Input: dimensioned drawing with shaded views. Units: mm. Origin: part minimum x, y, z. A direction names the side the tool comes from. Give positions to 0.01 mm unless a question says otherwise; leave off trailing zeros. Order: outer loops, then holes, each group sorted by start corner. A loop starts at its lowest first (then second) coordinate and runs counter-clockwise, first axis right, second up. Notation, with made-up numbers: M 81,3.25 L 86,3.25 A11 ccw 86,12.25 Z; hole C 65,86.5 d4. An arc over 180 degrees is marked long. Answer in a Markdown table with one row per item. Add a question column.
(1) Section query C-C, the plane z = 14. Return loops of the section in (x, y), plus the area to 3 significant figures.
(2) Pin query (flat end, axial travel): P1, Ø4, axis at x = 49.5, z = 19.5, coming from the +Y side; P2, Ø2.5, axis at x = 57.63, y = 57.63, coming from the -Z side; P3, Ø1.9, axis at y = 5, z = 29, coming from the +X side; P4, Ø5, axis at y = 66.5, z = 27, coming from the +X side (1 decimal). Return the tip coordinate at first contact, or that it passes through.
(3) Material intervals for line 1 along Y through (x, z) = (34, 8) (1 decimal); line 2 along Y through (x, z) = (46, 7.5) (1 decimal); line 3 along X through (y, z) = (47, 25.5), sorted ascending.
(4) Mould query, pull axis Y, two halves, no side actions, for the marked faces 4, 5 and 6. Classes: pulls with the +Y half, pulls with the -Y half, needs draft (parallel to the pull), parting line crosses it, or undercut.
(5) Section query A-A, the plane y = 35. Return loops of the section in (x, z), plus the area to 3 significant figures.
(6) Set-up query: the marked faces 1, 2 and 3. Return all of +Z, -Z, +X, -X, +Y, -Y with unobstructed straight access to the full face (end or side cutting, diameter ignored); none if empty.
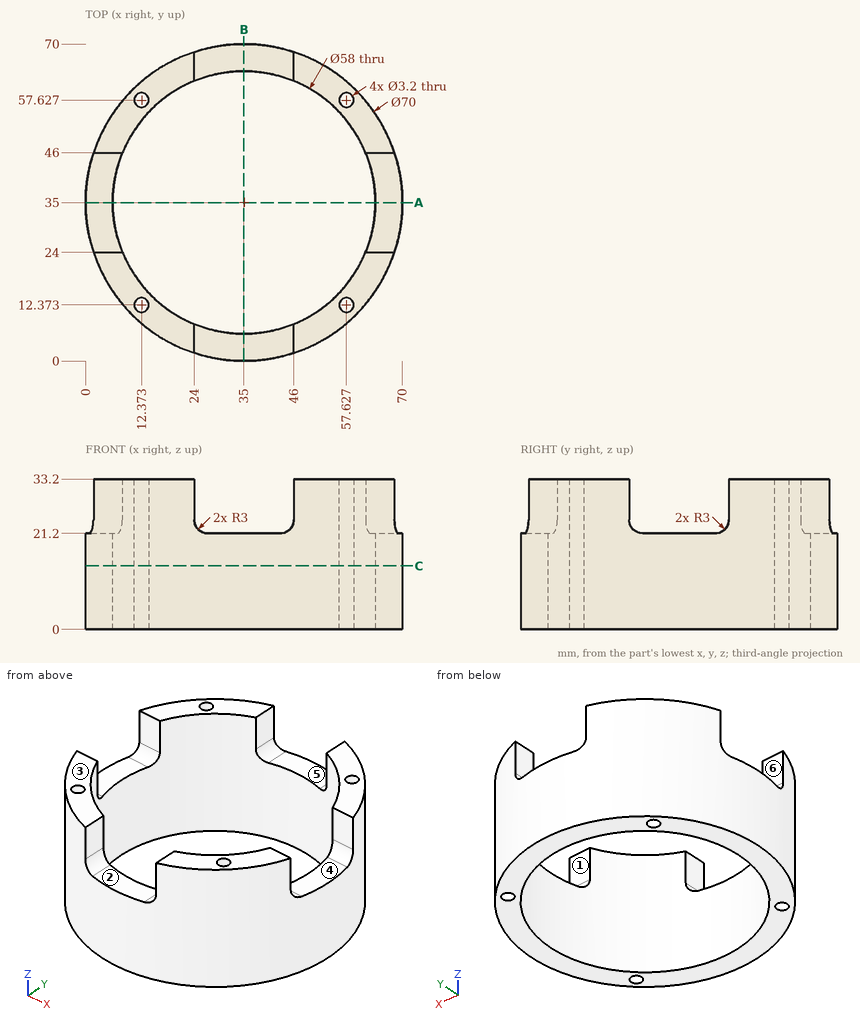
Values follow:
| question | item | result |
|---|---|---|
| 1 | outline | C 35,35 d70; hole C 35,35 d58; hole C 12.37,12.37 d3.2; hole C 12.37,57.63 d3.2; hole C 57.63,12.37 d3.2; hole C 57.63,57.63 d3.2 |
| 1 | area | 1,170 mm² |
| 2 | P1 | stops at y = 67.69 |
| 2 | P2 | passes through |
| 2 | P3 | stops at x = 54.52 |
| 2 | P4 | stops at x = 54.6 |
| 3 | line 1 | y = 0 to 6, 64 to 70 |
| 3 | line 2 | y = 1.8 to 8.2, 61.8 to 68.2 |
| 3 | line 3 | x = 2.12 to 8.6, 61.4 to 67.88 |
| 4 | face 4 | undercut |
| 4 | face 5 | needs draft |
| 4 | face 6 | undercut |
| 5 | outline | M 0,0 L 6,0 L 6,21.2 L 0,21.2 Z; M 64,0 L 70,0 L 70,21.2 L 64,21.2 Z |
| 5 | area | 254 mm² |
| 6 | face 1 | +Z, +X, -X |
| 6 | face 2 | +Z, +Y, -Y |
| 6 | face 3 | +Z, +X, -X, +Y, -Y |
